The model under review builds one solid part; all positions refer to its coordinate system, in mm. A direction names the side the tool comes from. Coordinates: 2 decimals unless noted, no trailing zeros. Order: outer loops, then holes, each group sorted by start corner. A loop starts at its lowest first (then second) coordinate and runs counter-clockwise, first axis right, second up. Notation, with made-up numbers: M 2,-31.75 L 15,-31.75 A32 cw 15,-4.75 Z; hole C -37.75,56 d11. An arc over 180 degrees is marked long. Write each question's results on one line, items separated by ' | '.
Autodesk Inventor part; units mm, degrees
ref_plane "YZ Plane" through (0, 0, 0) normal (1, 0, 0) x (0, 1, 0)
ref_plane "XZ Plane" through (0, 0, 0) normal (0, 1, 0) x (-1, 0, 0)
ref_plane "XY Plane" through (0, 0, 0) normal (0, 0, 1) x (1, 0, 0)
sketch "スケッチ1" plane through (0, 0, 0) normal (0, 0, 1) x (1, 0, 0)
  line L0 (-9, -22.5) -> (9, -22.5)
  line L1 (9, -22.5) -> (9, 22.5)
  line L2 (9, 22.5) -> (-9, 22.5)
  line L3 (-9, 22.5) -> (-9, -22.5)
  line L4 (-9, -22.5) -> (9, 22.5) construction
  line L5 (9, -22.5) -> (-9, 22.5) construction
  point P0 (0, 0)
  dimension "d0" = 18
  dimension "d1" = 45
extrude "押し出し1" add sketch "スケッチ1" along normal blind 10
sketch "スケッチ2" plane through (0, 0, 10) normal (0, 0, 1) x (1, 0, 0)
  line L0 (-9, 22.5) -> (-9, -22.5)
  line L1 (-9, -22.5) -> (-9, 2.1)
  line L2 (-9, 2.1) -> (9, 2.1)
  line L3 (9, -22.5) -> (9, 22.5)
  line L4 (9, 2.1) -> (9, -22.5)
  line L5 (9, -22.5) -> (6.25, -22.5)
  line L6 (-9, -22.5) -> (9, -22.5)
  line L7 (6.25, -22.5) -> (6.25, 0.1)
  line L8 (6.25, 0.1) -> (-6.25, 0.1)
  line L9 (-6.25, 0.1) -> (-6.25, -22.5)
  line L10 (-9, -22.5) -> (-6.25, -22.5)
  point P0 (0, 0)
  dimension "d4" = 12.5
  dimension "d5" = 2.75
  dimension "d6" = 22.6
  dimension "d7" = 2
extrude "押し出し2" add sketch "スケッチ2" along normal blind 3 contours L2 L3 L5 L7 L8 L9 L6 L0
sketch "スケッチ3" plane through (0, 0, 10) normal (0, 0, 1) x (1, 0, 0)
  circle A0 centre (0, 18.5) radius 1.5
  line L0 (9, 22.5) -> (-9, 22.5)
  point P0 (0, 0)
  dimension "d10" = 3
  dimension "d11" = 4
extrude "押し出し3" cut sketch "スケッチ3" against normal through all
sketch "スケッチ4" plane through (-9, -22.5, 0) normal (0, -1, 0) x (1, 0, 0)
  circle A0 centre (9, 5) radius 1.5
  line L0 (18, 0) -> (18, 13)
  line L1 (0, 0) -> (18, 0)
  point P0 (9, 0)
  dimension "d14" = 3
  dimension "d15" = 9
  dimension "d16" = 5
extrude "押し出し4" cut sketch "スケッチ4" against normal blind 25
properties part number "ジョイントモーター付き"
1) Take a section at C-C on y = 18.5. State the section outline as (x, z) points.
Solutions:
outline: M -9,0 L -1.5,0 L -1.5,10 L -9,10 Z; M 1.5,0 L 9,0 L 9,10 L 1.5,10 Z
2) Take a section at A-A on z = 5. State the section outline as (x, y) points, plus the area to 3 significant figures.
Solutions:
outline: M -9,-22.5 L -1.5,-22.5 L -1.5,2.5 L 1.5,2.5 L 1.5,-22.5 L 9,-22.5 L 9,22.5 L -9,22.5 Z; hole C 0,18.5 d3 | area: 728 mm2
3) For faces 5 (the cylindrical face through (0, 20, 5)), 6 (the flat face through (0, 12, 10)), 7 (the flat face through (0, 0.1, 11)), list the 3-axis set-ups (+Z, -Z, +X, -X, +Y, -Y) from which the entire face can be reached by the end or side of a thin tool; tool diameter is ignored.
Solutions:
face 5: +Z, -Z | face 6: +Z, +X, -X, +Y | face 7: +Z, -Y
4) Take a section at D-D on x = 4. State the section outline as (y, z) points.
Solutions:
outline: M -22.5,0 L 22.5,0 L 22.5,10 L 2.1,10 L 2.1,13 L 0.1,13 L 0.1,10 L -22.5,10 Z
5) For pin 1 (1 mm diameter, centred on x = -4, y = -13.5, fed in from +Z); pin 2 (1.5 mm diameter, centred on x = -1.5, z = 12, fed in from -Y); pin 3 (2.5 mm diameter, centred on x = 2, z = 12, fed in from +Y), all flat-tipped, find the tip position at first contact; note any pin that passes through.
Solutions:
pin 1: z = 10 | pin 2: y = 0.1 | pin 3: y = 2.1
6) The part is to be moulded in two halves that separate along Z. For faces 1 (the cylindrical face through (-1.5, -10.18, 5.07)), 2 (the flat face through (0, 2.5, 5)), 3 (the flat face through (6.25, -11, 11)), 4 (the flat face through (0, 0, 0)), say which applies: pulls with the +Z half, pulls with the -Z half, needs draft (parallel to the pull), parting line crosses it, or undercut.
Solutions:
face 1: undercut | face 2: undercut | face 3: needs draft | face 4: pulls with the -Z half
7) Take a section at B-B on x = 0. State the section outline as (y, z) points, plus the area to 3 significant figures.
Solutions:
outline: M -22.5,0 L 17,0 L 17,10 L 2.1,10 L 2.1,13 L 0.1,13 L 0.1,10 L -22.5,10 L -22.5,6.5 L 2.5,6.5 L 2.5,3.5 L -22.5,3.5 Z; M 20,0 L 22.5,0 L 22.5,10 L 20,10 Z | area: 351 mm2
8) To check wall thickness, follow line 1 along Z through (x, y) = (0, -16.5); line 2 along Y through (x, z) = (0, 5.75); line 3 along X through (y, z) = (-19, 6.25). State the ranges of each line that lie inside material, in increasing order.
Solutions:
line 1: 0 to 3.5, 6.5 to 10 | line 2: 2.5 to 17, 20 to 22.5 | line 3: -9 to -0.83, 0.83 to 9
